Source: three-view drawing plus pictorial views. Frame: mm from the lowest corner of the part. Round coordinates to 2 decimals unless told otherwise and drop trailing zeros. Order: outer loops, then holes, each group sorted by start corner. A loop starts at its lowest first (then second) coordinate and runs counter-clockwise, first axis right, second up. Notation, with made-up numbers: M 62.5,-39.75 L 66.5,-39.75 A32 ccw 66.5,-8.75 Z; hole C -14,85 d7. An arc over 180 degrees is marked long. Return JSON: item names as keys, results as strings. Group by question number.
Q1. Ray query, probe 1 along X at (y, z) = (2, 11); probe 2 along Z at (x, y) = (9.5, 3); probe 3 along X at (y, z) = (5.5, 8.5). Return the intervals inside material, ascending.
Q2. Cut plane A-A on x = 11. Output: boundary loops of the cut face in (y, z).
Q3. Cut plane B-B on z = 11. Output: boundary loops of the cut face in (x, y).
Q4. Contact query for flat-ended pins moving along their axis: pin 1 (4 mm diameter, centred on y = 10.5, z = 2.5, fed in from -X); pin 2 (0.6 mm diameter, centred on x = 11, z = 2, fed in from +Y); pin 3 (4 mm diameter, centred on y = 7, z = 3.5, fed in from +X). Output: stop coordinate, or through.
Q5. Cut plane C-C on y = 5.25. Output: boundary loops of the cut face in (x, z), and give its area (3 significant figures).
Q6. Mould query, pull axis Z, two halves, no side actions, for the marked faces 1, 2 and 3. Classes: released by +Z, released by -Z, zero draft, split by the parting line, or undercut.
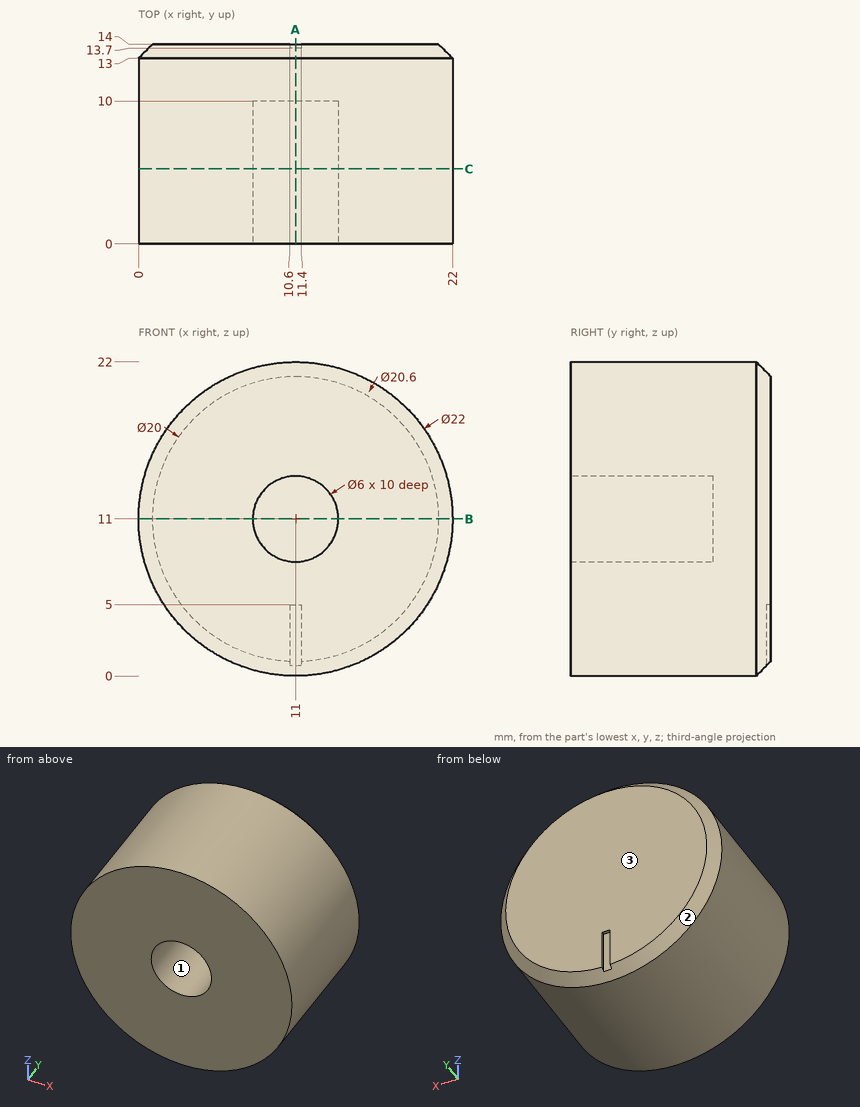
Result sheet:
{
 "1": {"probe 1": "x = 0 to 8, 14 to 22", "probe 2": "z = 0.1 to 8.4, 13.6 to 21.9", "probe 3": "x = 0.29 to 9.34, 12.66 to 21.71"},
 "2": {"outline": "M 0,0 L 13,0 L 13.7,0.7 L 13.7,5 L 14,5 L 14,21 L 13,22 L 0,22 L 0,14 L 10,14 L 10,8 L 0,8 Z"},
 "3": {"outline": "M 0,0 L 8,0 L 8,10 L 14,10 L 14,0 L 22,0 L 22,13 L 21,14 L 1,14 L 0,13 Z"},
 "4": {"pin 1": "stops at x = 2.13", "pin 2": "stops at y = 13.7", "pin 3": "stops at x = 20.53"},
 "5": {"outline": "C 11,11 d22; hole C 11,11 d6", "area": "352 mm²"},
 "6": {"face 1": "undercut", "face 2": "split by the parting line", "face 3": "zero draft"}
}
